Can you work these out from the model? Positions are in its coordinate system, mm. A direction names the side the tool comes from. Give positions to 0.01 mm unless a question says otherwise; leave off trailing zeros. Order: outer loops, then holes, each group sorted by start corner. A loop starts at its lowest first (then second) coordinate and runs counter-clockwise, first axis right, second up. Notation, with made-up numbers: M -37.75,6.25 L -6.75,6.25 A19 ccw -6.75,27.25 Z; hole C 22,16.5 d6. An arc over 180 degrees is marked long. Use one line per item in the form item = value. Start each with the question number.
1. We'd pull the mould along Y, two halves only. Please class faces 1 (the face through (25, -26, -44.45)), 2 (the face through (-26.723, -47.669, 35.474)), 3 (the face through (26, 44.45, 26)), 4 (the face through (44.45, 25, 26)): +Y half, -Y half, draft (parallel to the pull), parting line (faces both ways), or undercut.
2. I want a section at D-D, the plane z = 0. List the corners of the cut face in (x, y) for me.
3. For faces 5 (the face through (0, 0, 44.45)), 6 (the face through (0, -44.45, 0)), 7 (the face through (-26, 25, -44.45)), 8 (the face through (44.45, -26, -25)), which set-ups out of +Z, -Z, +X, -X, +Y, -Y let a thin tool reach every point of the face, with its end or its side?
4. I need wall thicknesses on L1, parallel to Y at x = -25.4, z = -46.75; L2, parallel to X at y = 25, z = -46. Which ranges of each line are inside material? Lowest first, please.
5. Will these pins go through, and if not, where does the flat tip stop? P1, Ø12, axis at x = -25.4, y = 0, coming from the -Z side; P2, Ø12, axis at y = -25.4, z = -25.4, coming from the -X side; P3, Ø3, axis at y = 22, z = -20.5, coming from the +X side.
6. I want a section at C-C, the plane y = 25.4. List the corners of the cut face in (x, z) for me.
Autodesk Fusion 360 part; units mm, degrees
sketch "Sketch1" plane through (0, 0, 0) normal (0, 0, 1) x (1, 0, 0)
  line L0 (50.8, -50.8) -> (-50.8, -50.8)
  line L1 (-50.8, -50.8) -> (-50.8, 50.8)
  line L2 (-50.8, 50.8) -> (50.8, 50.8)
  line L3 (50.8, 50.8) -> (50.8, -50.8)
  line L4 (50.8, -50.8) -> (-50.8, 50.8) construction
  line L5 (-50.8, -50.8) -> (50.8, 50.8) construction
  dimension "d1" = 101.6
  dimension "d2" = 101.6
extrude "Extrude1" add sketch "Sketch1" along normal mid plane 101.6
sketch "Sketch2" plane through (0, 0, 50.8) normal (0, 0, 1) x (-1, 0, 0)
  line L0 (-50.8, -50.8) -> (50.8, -50.8)
  line L1 (50.8, -50.8) -> (50.8, 50.8)
  line L2 (50.8, 50.8) -> (-50.8, 50.8)
  line L3 (-50.8, 50.8) -> (-50.8, -50.8)
  circle A0 centre (0, 0) radius 10.16
  dimension "d5" = 20.32
extrude "Extrude2" cut sketch "Sketch2" against normal blind 6.35 contours A0
sketch "Sketch3" plane through (0, -50.8, 0) normal (0, -1, 0) x (1, 0, 0)
  line L0 (50.8, -50.8) -> (50.8, 50.8)
  line L1 (50.8, 50.8) -> (-50.8, 50.8)
  line L2 (-50.8, 50.8) -> (-50.8, -50.8)
  line L3 (-50.8, -50.8) -> (50.8, -50.8)
  line L4 (-50.8, 50.8) -> (50.8, -50.8) construction
  line L5 (50.8, 50.8) -> (-50.8, -50.8) construction
  circle A0 centre (0, 0) radius 10.16
  circle A1 centre (-25.4, 25.4) radius 10.16
  circle A2 centre (25.4, -25.4) radius 10.16
  dimension "d9" = 20.32
  dimension "d12" = 20.32
  dimension "d13" = 20.32
extrude "Extrude3" cut sketch "Sketch3" against normal blind 6.35 contours A0 | A1 | A2
sketch "Sketch4" plane through (50.8, 0, 0) normal (1, 0, 0) x (0, 1, 0)
  line L0 (50.8, -50.8) -> (50.8, 50.8)
  line L1 (50.8, 50.8) -> (-50.8, 50.8)
  line L2 (-50.8, 50.8) -> (-50.8, -50.8)
  line L3 (-50.8, -50.8) -> (50.8, -50.8)
  line L4 (-50.8, 50.8) -> (50.8, -50.8) construction
  line L5 (50.8, 50.8) -> (-50.8, -50.8) construction
  circle A0 centre (0, 0) radius 10.16
  circle A1 centre (25.4, 25.4) radius 10.16
  circle A2 centre (25.4, -25.4) radius 10.16
  circle A3 centre (-25.4, -25.4) radius 10.16
  circle A4 centre (-25.4, 25.4) radius 10.16
  dimension "d16" = 20.32
  dimension "d17" = 20.32
  dimension "d18" = 20.32
  dimension "d19" = 20.32
  dimension "d20" = 20.32
extrude "Extrude4" cut sketch "Sketch4" against normal blind 6.35 contours A0 | A1 | A2 | A3 | A4
sketch "Sketch5" plane through (0, 50.8, 0) normal (0, 1, 0) x (-1, 0, 0)
  line L0 (50.8, -50.8) -> (50.8, 50.8)
  line L1 (50.8, 50.8) -> (-50.8, 50.8)
  line L2 (-50.8, 50.8) -> (-50.8, -50.8)
  line L3 (-50.8, -50.8) -> (50.8, -50.8)
  circle A0 centre (-25.4, 25.4) radius 10.16
  circle A1 centre (25.4, 25.4) radius 10.16
  circle A2 centre (25.4, -25.4) radius 10.16
  circle A3 centre (-25.4, -25.4) radius 10.16
  dimension "d26" = 20.32
extrude "Extrude5" cut sketch "Sketch5" against normal blind 6.35 contours A0 | A1 | A2 | A3
sketch "Sketch6" plane through (-50.8, 0, 0) normal (-1, 0, 0) x (0, -1, 0)
  line L0 (50.8, -50.8) -> (50.8, 50.8)
  line L1 (50.8, 50.8) -> (-50.8, 50.8)
  line L2 (-50.8, 50.8) -> (-50.8, -50.8)
  line L3 (-50.8, -50.8) -> (50.8, -50.8)
  circle A0 centre (-25.4, 25.4) radius 10.16
  circle A1 centre (25.4, -25.4) radius 10.16
  dimension "d29" = 20.32
  dimension "d30" = 20.32
extrude "Extrude6" cut sketch "Sketch6" against normal blind 6.35 contours A0 | A1
sketch "Sketch7" plane through (0, 0, -50.8) normal (0, 0, -1) x (1, 0, 0)
  line L0 (-50.8, -50.8) -> (50.8, -50.8)
  line L1 (50.8, -50.8) -> (50.8, 50.8)
  line L2 (50.8, 50.8) -> (-50.8, 50.8)
  line L3 (-50.8, 50.8) -> (-50.8, -50.8)
  circle A0 centre (-25.4, 0) radius 10.16
  circle A1 centre (-25.4, -25.4) radius 10.16
  circle A2 centre (-25.4, 25.4) radius 10.16
  circle A3 centre (25.4, 25.4) radius 10.16
  circle A4 centre (25.4, 0) radius 10.16
  circle A5 centre (25.4, -25.4) radius 10.16
  dimension "d33" = 20.32
extrude "Extrude7" cut sketch "Sketch7" against normal blind 6.35 contours A0 | A1 | A2 | A3 | A4 | A5
fillet "Fillet1" radius 2.032 12 edges at (50.8, 0, 50.8) (0, 50.8, 50.8) (-50.8, 0, 50.8) (0, -50.8, 50.8) (-50.8, -50.8, 0) (50.8, -50.8, 0) (50.8, 50.8, 0) (-50.8, 50.8, 0) (0, 50.8, -50.8) (50.8, 0, -50.8) (0, -50.8, -50.8) (-50.8, 0, -50.8)
equation "d1 = dicesize"
equation "d2 = dicesize"
equation "d3 = dicesize / 2"
equation "d5 = DivotDia"
equation "d6 = ( -1 / 4 ) * 1 in"
equation "d9 = DivotDia"
equation "d12 = DivotDia"
equation "d13 = DivotDia"
equation "d14 = ( -1 / 4 ) * 1 in"
equation "d16 = DivotDia"
equation "d17 = DivotDia"
equation "d18 = DivotDia"
equation "d19 = DivotDia"
equation "d20 = DivotDia"
equation "d21 = ( -1 / 4 ) * 1 in"
equation "dicesize = 4 in"
equation "DivotDia = 0.8 in"
equation "DivotDepth = 0.25 in"
equation "d26 = DivotDia"
equation "d29 = DivotDia"
equation "d30 = DivotDia"
equation "d33 = DivotDia"
Check result:
q1.face_1 = undercut
q1.face_2 = draft
q1.face_3 = +Y half
q1.face_4 = undercut
q2.outline = M -50.8,-48.77 A2.03 ccw -48.77,-50.8 L -10.16,-50.8 L -10.16,-44.45 L 10.16,-44.45 L 10.16,-50.8 L 48.77,-50.8 A2.03 ccw 50.8,-48.77 L 50.8,-10.16 L 44.45,-10.16 L 44.45,10.16 L 50.8,10.16 L 50.8,48.77 A2.03 ccw 48.77,50.8 L -48.77,50.8 A2.03 ccw -50.8,48.77 Z
q3.face_5 = +Z
q3.face_6 = -Y
q3.face_7 = -Z
q3.face_8 = +X
q4.L1 = -50.8 to -35.56, -15.24 to -10.16, 10.16 to 15.24, 35.56 to 50.8
q4.L2 = -50.8 to -35.55, -15.25 to 15.25, 35.55 to 50.8
q5.P1 = -44.45
q5.P2 = -44.45
q5.P3 = 44.45
q6.outline = M -50.8,-48.77 A2.03 ccw -48.77,-50.8 L -35.56,-50.8 L -35.56,-44.45 L -15.24,-44.45 L -15.24,-50.8 L 15.24,-50.8 L 15.24,-44.45 L 35.56,-44.45 L 35.56,-50.8 L 48.77,-50.8 A2.03 ccw 50.8,-48.77 L 50.8,-35.56 L 44.45,-35.56 L 44.45,-15.24 L 50.8,-15.24 L 50.8,15.24 L 44.45,15.24 L 44.45,35.56 L 50.8,35.56 L 50.8,48.77 A2.03 ccw 48.77,50.8 L -48.77,50.8 A2.03 ccw -50.8,48.77 L -50.8,35.56 L -44.45,35.56 L -44.45,15.24 L -50.8,15.24 Z
